Read the model definition and answer for the solid it produces. Units are mm, in the model's axes. Face numbers are marked on the shaded views. A direction names the side the tool comes from. Coordinates: 2 decimals unless noted, no trailing zeros. Order: outer loops, then holes, each group sorted by start corner. A loop starts at its lowest first (then second) coordinate and runs counter-clockwise, first axis right, second up. Notation, with made-up numbers: (-9, -2) -> (41, -2) arc R15 ccw to (41, 18) -> close; hole circle Ø5 at (33, 15). An arc over 180 degrees is marked (long way). Answer as a JSON object with one key per item and string values. Group by question number.
1) Section D-D on y = -10 is taken. Determine the outline of the cut face in (x, z), and give its area (3 significant figures).
2) Consider L1, parallel to Z at x = -75.5, y = -10; L2, parallel to Y at x = -77.75, z = 39; L3, parallel to Y at x = -76.35, z = 39. Determine where each line is inside the solid, lowest interval first.
3) Section A-A on x = -77.5 is taken. Determine the outline of the cut face in (y, z), and give its area (3 significant figures).
4) Section B-B on z = 69 is taken. Determine the outline of the cut face in (x, y), and give its area (3 significant figures).
5) Section C-C on y = 20 is taken. Determine the outline of the cut face in (x, z).
6) A tool of negligible diameter and unlimited length cuts with its end or side. For the marked faces 1 and 2, from which of +Z, -Z, +X, -X, +Y, -Y can it reach the whole face along a straight path? Write none if from no direction.
7) Given pin 1 (6 mm diameter, centred on y = -6.5, z = 71, fed in from +X); pin 2 (1.5 mm diameter, centred on x = -78, z = 57, fed in from +Y); pin 3 (4 mm diameter, centred on y = 13.5, z = 53, fed in from +X), each flat-ended and moving along its own axis, determine where each tip first touches the part or whether it passes through.
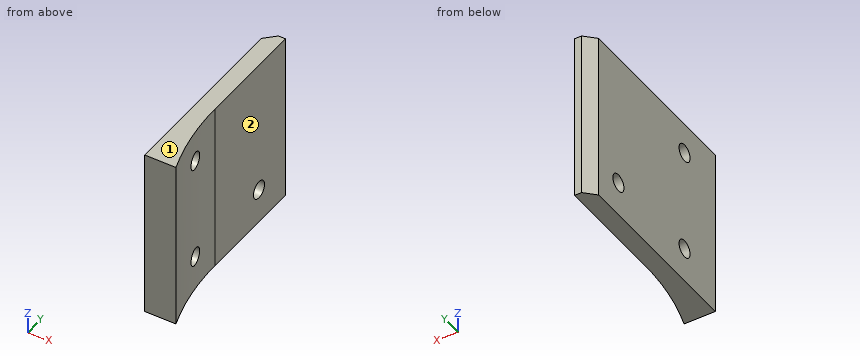
from build123d import *

# Parameters (mm, degrees)
BOX750_W           = 148
BOX750_H           = 74
BOX750_DEPTH       = 55
CYLINDER1790_R     = 74
CYLINDER1790_DEPTH = 60
CYLINDER1795_R     = 2.5
CYLINDER1795_DEPTH = 40
CYLINDER1791_R     = 2.5
CYLINDER1791_DEPTH = 40
CYLINDER1794_R     = 2.5
CYLINDER1794_DEPTH = 40
BOX755_W           = 10
BOX755_H           = 56
BOX755_DEPTH       = 49
CHAMFER061_SIZE    = 3


with BuildPart() as krychle750:
    # Box750 → Box750 (new body)
    with BuildSketch(Plane(origin=(-74, 0, 29), x_dir=(1, 0, 0), z_dir=(0, 0, 1))):
        with Locations((74, 37)):
            Rectangle(BOX750_W, BOX750_H)
    extrude(amount=BOX750_DEPTH)


with BuildPart() as obj1:
    # Cylinder1790 → Cylinder1790 (new body)
    with BuildSketch(Plane.XY.offset(26)):
        Circle(CYLINDER1790_R)
    extrude(amount=CYLINDER1790_DEPTH)


with BuildPart() as obj2:
    # Cylinder1795 → Cylinder1795 (new body)
    with BuildSketch(Plane(origin=(-86, 20, 39), x_dir=(0, 0, -1), z_dir=(1, 0, 0))):
        Circle(CYLINDER1795_R)
    extrude(amount=CYLINDER1795_DEPTH)


with BuildPart() as obj3:
    # Cylinder1791 → Cylinder1791 (new body)
    with BuildSketch(Plane(origin=(-86, -10, 69), x_dir=(0, 0, -1), z_dir=(1, 0, 0))):
        Circle(CYLINDER1791_R)
    extrude(amount=CYLINDER1791_DEPTH)


with BuildPart() as compound910:
    # Cylinder1794 → Cylinder1794 (new body)
    with BuildSketch(Plane(origin=(-86, -10, 39), x_dir=(0, 0, -1), z_dir=(1, 0, 0))):
        Circle(CYLINDER1794_R)
    extrude(amount=CYLINDER1794_DEPTH)

    # Compound910: union obj2, obj3
    add(obj2.part)
    add(obj3.part)


with BuildPart() as cut551:
    # Box755 → Box755 (new body)
    with BuildSketch(Plane(origin=(-79, -24, 29), x_dir=(1, 0, 0), z_dir=(0, 0, 1))):
        with Locations((5, 28)):
            Rectangle(BOX755_W, BOX755_H)
    extrude(amount=BOX755_DEPTH)

    # Chamfer061
    chamfer061_edges = [cut551.edges().sort_by_distance(p)[0] for p in [
        (-79, 32, 53.5),
    ]]
    chamfer(chamfer061_edges, length=CHAMFER061_SIZE)

    # Cut549: cut Compound910
    add(compound910.part, mode=Mode.SUBTRACT)

    # Cut550: cut obj1
    add(obj1.part, mode=Mode.SUBTRACT)

    # Cut551: cut Krychle750
    add(krychle750.part, mode=Mode.SUBTRACT)


solid = cut551.part
Worked answers:
{
 "1": {"outline": "(-79, 29) -> (-73.32, 29) -> (-73.32, 36.5) -> (-79, 36.5) -> close; (-79, 41.5) -> (-73.32, 41.5) -> (-73.32, 66.5) -> (-79, 66.5) -> close; (-79, 71.5) -> (-73.32, 71.5) -> (-73.32, 78) -> (-79, 78) -> close", "area": "221 mm²"},
 "2": {"L1": "z = 29 to 36.5, 41.5 to 66.5, 71.5 to 78", "L2": "y = -24 to -12.5, -7.5 to 17.5, 22.5 to 30.25", "L3": "y = -24 to -12.5, -7.5 to 17.5, 22.5 to 31.65"},
 "3": {"outline": "(-24, 29) -> (30.5, 29) -> (30.5, 78) -> (-24, 78) -> close; hole circle Ø5 at (-10, 39); hole circle Ø5 at (-10, 69); hole circle Ø5 at (20, 39)", "area": "2,610 mm²"},
 "4": {"outline": "(-79, -24) -> (-70, -24) arc R74 cw to (-72.94, -12.5) -> (-79, -12.5) -> close; (-79, -7.5) -> (-73.62, -7.5) arc R74 cw to (-74, 0) -> (-74, 32) -> (-76, 32) -> (-79, 29) -> close", "area": "279 mm²"},
 "5": {"outline": "(-79, 29) -> (-74, 29) -> (-74, 36.5) -> (-79, 36.5) -> close; (-79, 41.5) -> (-74, 41.5) -> (-74, 78) -> (-79, 78) -> close"},
 "6": {"face 1": "+Z, +X, -X, +Y, -Y", "face 2": "+Z, -Z, +X, +Y"},
 "7": {"pin 1": "stops at x = -73.39", "pin 2": "stops at y = 30.75", "pin 3": "stops at x = -74"}
}
